Autodesk Inventor part; units mm, degrees
ref_plane "YZ Plane" through (0, 0, 0) normal (1, 0, 0) x (0, 1, 0)
ref_plane "XZ Plane" through (0, 0, 0) normal (0, 1, 0) x (-1, 0, 0)
ref_plane "XY Plane" through (0, 0, 0) normal (0, 0, 1) x (1, 0, 0)
sketch "Drawing" plane through (0, 0, 0) normal (0, 0, 1) x (1, 0, 0)
  line L0 (-58.5227, 93.5052) -> (128.141, 93.5052) construction
  line L1 (128.141, 93.5052) -> (128.141, -71.3811) construction
  line L2 (128.141, -71.3811) -> (-58.5227, -71.3811) construction
  line L3 (-58.5227, -71.3811) -> (-58.5227, 93.5052) construction
  line L4 (-58.5227, 93.5052) -> (-58.5227, 50)
  line L5 (-54.9683, 50) -> (-54.9683, -50)
  line L6 (-58.5227, 50) -> (-54.9683, 50)
  line L7 (0, 0) -> (-54.9683, 0) construction
  line L8 (0, 0) -> (0, 93.5052) construction
  line L9 (0, 93.5052) -> (0, -71.3811)
  line L10 (-58.5227, 0) -> (128.141, 0)
  circle A0 centre (23, 22.25) radius 2.5
  circle A1 centre (23, 22.25) radius 1.5
  circle A2 centre (20, 35) radius 1.75
  dimension "d16" = 164.8863
  dimension "d20" = 3.5544
  dimension "d21" = 100
  dimension "d22" = 43.5052
  dimension "d48" = 5
  dimension "d49" = 1
  dimension "d50" = 3.5
sketch "Sketch2" plane through (0, 0, 0) normal (0, 0, 1) x (1, 0, 0)
  line L0 (28, 50) -> (-28, 50)
  line L1 (-34, 44) -> (-34, -44)
  line L2 (-28, -50) -> (28, -50)
  line L3 (34, -44) -> (34, 44)
  line L4 (34, 50) -> (-34, -50) construction
  line L5 (-34, 50) -> (34, -50) construction
  arc A0 (-28, 50) -> (-34, 44) centre (-28, 44) ccw
  arc A1 (34, 44) -> (28, 50) centre (28, 44) ccw
  arc A2 (-34, -44) -> (-28, -50) centre (-28, -44) ccw
  arc A3 (28, -50) -> (34, -44) centre (28, -44) ccw
  line L6 (28.5085, 38) -> (28.519, 38)
  line L7 (28.0455, -38) -> (28.5, -38)
  line L8 (-58.5227, 0) -> (128.141, 0)
  line L9 (0, 0) -> (0, 93.5052) construction
  line L10 (0, 93.5052) -> (0, -71.3811)
  line L11 (22, 44) -> (22, 44.5)
  line L12 (30.5, 36) -> (30.5, -36)
  line L13 (22.0455, -44) -> (22.0455, -44.5)
  line L14 (-22.0163, -44.039) -> (-22.0163, -44.5)
  line L15 (-30.5, -36.039) -> (-30.5, 36)
  line L16 (-22, 44) -> (-22, 44.5)
  arc A4 (-28, 38) -> (-22, 44) centre (-28, 44) ccw
  arc A5 (22, 44) -> (28, 38) centre (28, 44) ccw
  arc A6 (28.0455, -38) -> (22.0455, -44) centre (28.0455, -44) ccw
  arc A7 (-22.0163, -44.039) -> (-28.0163, -38.039) centre (-28.0163, -44.039) ccw
  arc A8 (-22.0163, -44.5) -> (-20.0163, -46.5) centre (-20.0163, -44.5) ccw
  arc A9 (-30.5, -36.039) -> (-28.5, -38.039) centre (-28.5, -36.039) ccw
  arc A10 (20.0455, -46.5) -> (22.0455, -44.5) centre (20.0455, -44.5) ccw
  arc A11 (28.5, -38) -> (30.5, -36) centre (28.5, -36) ccw
  arc A12 (30.5, 36) -> (28.5, 38) centre (28.5, 36) ccw
  arc A13 (22, 44.5) -> (20, 46.5) centre (20, 44.5) ccw
  arc A14 (-28.5, 38) -> (-30.5, 36) centre (-28.5, 36) ccw
  arc A15 (-20, 46.5) -> (-22, 44.5) centre (-20, 44.5) ccw
  circle A16 centre (23, 22.25) radius 2.5
  circle A17 centre (23, 22.25) radius 1.5
  circle A18 centre (20, 35) radius 1.75
  circle A19 centre (-23, 22.25) radius 2.5
  circle A20 centre (-23, 22.25) radius 1.5
  circle A21 centre (-20, 35) radius 1.75
  circle A22 centre (23, -22.25) radius 2.5
  circle A23 centre (23, -22.25) radius 1.5
  circle A24 centre (20, -35) radius 1.75
  circle A25 centre (-20, -35) radius 1.75
  circle A26 centre (-23, -22.25) radius 2.5
  circle A27 centre (-23, -22.25) radius 1.5
  circle A28 centre (-28, 44) radius 2
  circle A29 centre (28, 44) radius 2
  circle A30 centre (-28, -44) radius 2
  circle A31 centre (28, -44) radius 2
  circle A32 centre (0, 40) radius 2.5
  circle A33 centre (0, 40) radius 1.5
  circle A34 centre (0, -40) radius 2.5
  circle A35 centre (0, -40) radius 1.5
  line L17 (-20.0163, -46.5) -> (20.0455, -46.5)
  line L18 (22, 44.4601) -> (22, 44)
  line L19 (-28, 38) -> (-28.5, 38)
  line L20 (-20, 46.5) -> (20, 46.5)
  line L21 (-28.5, -38.039) -> (-28.5, -38.039)
  line L22 (28.5, 38) -> (28, 38)
  line L23 (-28.493, -38.1054) -> (-28.493, -38.1054)
  line L24 (-28.5, -38.039) -> (-28.0163, -38.039)
  line L25 (23.05, 44) -> (23.05, 44.5)
  arc A36 (23.05, 44.5) -> (20, 47.55) centre (20, 44.5) ccw
  line L26 (20, 47.55) -> (-20, 47.55)
  arc A37 (-20, 47.55) -> (-23.05, 44.5) centre (-20, 44.5) ccw
  line L27 (-23.05, 44.5) -> (-23.05, 44)
  arc A38 (-28, 39.05) -> (-23.05, 44) centre (-28, 44) ccw
  line L28 (-28, 39.05) -> (-28.5, 39.05)
  arc A39 (-28.5, 39.05) -> (-31.55, 36) centre (-28.5, 36) ccw
  line L29 (-31.55, 36) -> (-31.55, -36.039)
  arc A40 (-31.55, -36.039) -> (-28.5, -39.089) centre (-28.5, -36.039) ccw
  line L30 (-28.5, -39.089) -> (-28.0163, -39.089)
  arc A41 (-23.0663, -44.039) -> (-28.0163, -39.089) centre (-28.0163, -44.039) ccw
  line L31 (-23.0663, -44.039) -> (-23.0663, -44.5)
  arc A42 (-23.0663, -44.5) -> (-20.0163, -47.55) centre (-20.0163, -44.5) ccw
  line L32 (-20.0163, -47.55) -> (20.0455, -47.55)
  arc A43 (20.0455, -47.55) -> (23.0955, -44.5) centre (20.0455, -44.5) ccw
  line L33 (23.0955, -44.5) -> (23.0955, -44)
  arc A44 (28.0455, -39.05) -> (23.0955, -44) centre (28.0455, -44) ccw
  line L34 (28.0455, -39.05) -> (28.5, -39.05)
  arc A45 (28.5, -39.05) -> (31.55, -36) centre (28.5, -36) ccw
  line L35 (31.55, -36) -> (31.55, 36)
  arc A46 (31.55, 36) -> (28.5, 39.05) centre (28.5, 36) ccw
  line L36 (28.5, 39.05) -> (28, 39.05)
  arc A47 (23.05, 44) -> (28, 39.05) centre (28, 44) ccw
  line L37 (-33.5, -44) -> (-33.5, 44)
  arc A48 (-28, 49.5) -> (-33.5, 44) centre (-28, 44) ccw
  line L38 (-28, 49.5) -> (28, 49.5)
  arc A49 (33.5, 44) -> (28, 49.5) centre (28, 44) ccw
  line L39 (33.5, 44) -> (33.5, -44)
  arc A50 (28, -49.5) -> (33.5, -44) centre (28, -44) ccw
  line L40 (28, -49.5) -> (-28, -49.5)
  arc A51 (-33.5, -44) -> (-28, -49.5) centre (-28, -44) ccw
  point P0 (-34, 38)
  point P1 (34, 38)
  point P2 (-34, -38)
  point P3 (34, -38)
  point P4 (22, 50)
  point P5 (22, -50)
  point P6 (-34, 46.5)
  point P7 (34, -46.5)
  dimension "OuterWidth" = 68
  dimension "OuterLength" = 100
  dimension "d26" = 6
  dimension "d27" = 6
  dimension "d29" = 6
  dimension "d34" = 6
  dimension "d36" = 2
  dimension "d37" = 6
  dimension "d38" = 6
  dimension "d39" = 6
  dimension "d40" = 6
  dimension "d41" = 11
  dimension "d42" = 27.75
  dimension "d43" = 5
  dimension "d44" = 1
  dimension "d45" = 3.5
  dimension "d46" = 15
  dimension "d47" = 14
  dimension "d52" = 4
  dimension "d53" = 5
  dimension "d54" = 1
  dimension "d55" = 10
  dimension "d56" = 3.5
  dimension "d57" = 3.5
  dimension "d58" = 3.5
  dimension "d59" = 3.5
  dimension "d60" = 6
  dimension "d61" = 6
  dimension "d62" = 6
  dimension "d63" = 6
  dimension "d67" = 1.05
  dimension "d68" = 1.05
  dimension "d86" = 0.5
extrude "SideWalls" add sketch "Sketch2" along normal blind 35 contours A1 L3 L8 L39 A49 L38 L10 L0 | L10 L38 A48 L37 L8 L1 A0 L0 | L38 A49 L39 L8 L35 A46 L36 A47 L25 A36 L26 L10 | L10 L26 A37 L27 A38 L28 A39 L29 L8 L37 A48 L38 | L3 A3 L2 L10 L40 A50 L39 L8 | L26 A36 L25 A47 L36 A46 L35 L8 L12 A12 L6 L22 A5 L11 A13 L20 L10 | L10 L20 A15 L16 A4 L19 A14 L15 L8 L29 A39 L28 A38 L27 A37 L26 | L39 A50 L40 L10 L32 A43 L33 A44 L34 A45 L35 L8 | L8 L37 A51 L40 L10 L2 A2 L1 | L35 A45 L34 A44 L33 A43 L32 L10 L17 A10 L13 A6 L7 A11 L12 L8 | L8 L29 A40 L30 A41 L31 A42 L32 L10 L40 A51 L37 | L8 L15 A9 L24 A7 L14 A8 L17 L10 L32 A42 L31 A41 L30 A40 L29
extrude "GasketRingLower" add sketch "Sketch2" along normal blind 36.85 contours L26 A36 L25 A47 L36 A46 L35 L8 L12 A12 L6 L22 A5 L11 A13 L20 L10 | L10 L20 A15 L16 A4 L19 A14 L15 L8 L29 A39 L28 A38 L27 A37 L26 | L35 A45 L34 A44 L33 A43 L32 L10 L17 A10 L13 A6 L7 A11 L12 L8 | L8 L15 A9 L24 A7 L14 A8 L17 L10 L32 A42 L31 A41 L30 A40 L29
extrude "Bottom" add sketch "Sketch2" along normal blind 2.8 contours A1 L3 L8 L39 A49 L38 L10 L0 | L10 L38 A48 L37 L8 L1 A0 L0 | L38 A49 L39 L8 L35 A46 L36 A47 L25 A36 L26 L10 | L10 L26 A37 L27 A38 L28 A39 L29 L8 L37 A48 L38 | L3 A3 L2 L10 L40 A50 L39 L8 | L26 A36 L25 A47 L36 A46 L35 L8 L12 A12 L6 L22 A5 L11 A13 L20 L10 | L10 L20 A15 L16 A4 L19 A14 L15 L8 L29 A39 L28 A38 L27 A37 L26 | L39 A50 L40 L10 L32 A43 L33 A44 L34 A45 L35 L8 | L8 L37 A51 L40 L10 L2 A2 L1 | L20 A13 L11 A5 L22 A12 L6 L12 L8 L10 A32 | L10 A32 L8 L15 A14 L19 A4 L16 A15 L20 | L35 A45 L34 A44 L33 A43 L32 L10 L17 A10 L13 A6 L7 A11 L12 L8 | L8 L29 A40 L30 A41 L31 A42 L32 L10 L40 A51 L37 | A32 L10 A33 | L10 A33 A32 | L12 A11 L7 A6 L13 A10 L17 L10 A34 L8 | L8 L15 A9 L24 A7 L14 A8 L17 L10 L32 A42 L31 A41 L30 A40 L29 | A33 L10 | L10 A33 | L10 A34 L17 A8 L14 A7 L24 A9 L15 L8 | A34 L10 A35 | L10 A35 A34 | A35 L10 | L10 A35 | A16 | A17 | A18 | A19 | A20 | A21 | A22 | A23 | A24 | A25 | A26 | A27 | A28 | A29 | A30 | A31
extrude "PEMStuds" add sketch "Sketch2" along normal blind 6 contours A32 L10 A33 | L10 A33 A32 | A33 L10 | L10 A33 | A34 L10 A35 | L10 A35 A34 | A35 L10 | L10 A35 | A16 | A17 | A19 | A20 | A22 | A23 | A26 | A27
extrude "SmallerSupports" add sketch "Sketch2" along normal blind 4 contours A18 | A21 | A24 | A25
sketch "Sketch4" plane through (-23, -22.25, 6) normal (0, 0, 1) x (1, 0, 0)
  circle A0 centre (23, -17.75) radius 2.5
  circle A1 centre (46, 0) radius 2.5
  circle A2 centre (23, 62.25) radius 2.5
  circle A3 centre (0, 0) radius 2.5
  circle A4 centre (46, 44.5) radius 2.5
  circle A5 centre (-5, -21.75) radius 2
  circle A6 centre (51, -21.75) radius 2
  circle A7 centre (-5, 66.25) radius 2
  circle A8 centre (51, 66.25) radius 2
  circle A9 centre (0, 44.5) radius 2.5
  point P0 (23, 22.25)
  dimension "d101" = 17.75
  dimension "d102" = 23
hole "PEMStudHoles" at (0, -40, 6) at (23, -22.25, 6) at (0, 40, 6) at (-23, -22.25, 6) at (23, 22.25, 6) at (-23, 22.25, 6) direction (0, 0, -1) diameter 3 depth 4
hole "Hole2" at (28, 44, 6) at (-28, 44, 6) at (-28, -44, 6) at (28, -44, 6) direction (0, 0, -1) diameter 6 end through all both
ref_plane "Work Plane2" through (-32.2426, 48.2426, 35) normal (0, 0, 1) x (1, 0, 0)
sketch "Sketch6" plane through (-32.2426, 48.2426, 35) normal (0, 0, 1) x (1, 0, 0)
  line L0 (-1.2574, -92.2426) -> (-1.2574, -4.2426)
  arc A0 (4.2426, 1.2574) -> (-1.2574, -4.2426) centre (4.2426, -4.2426) ccw
  line L1 (4.2426, 1.2574) -> (60.2426, 1.2574)
  arc A1 (65.7426, -4.2426) -> (60.2426, 1.2574) centre (60.2426, -4.2426) ccw
  line L2 (65.7426, -4.2426) -> (65.7426, -92.2426)
  arc A2 (60.2426, -97.7426) -> (65.7426, -92.2426) centre (60.2426, -92.2426) ccw
  line L3 (60.2426, -97.7426) -> (4.2426, -97.7426)
  arc A3 (-1.2574, -92.2426) -> (4.2426, -97.7426) centre (4.2426, -92.2426) ccw
  line L4 (-1.7574, -4.2426) -> (-1.7574, -92.2426)
  arc A4 (-1.7574, -92.2426) -> (4.2426, -98.2426) centre (4.2426, -92.2426) ccw
  line L5 (4.2426, -98.2426) -> (60.2426, -98.2426)
  arc A5 (60.2426, -98.2426) -> (66.2426, -92.2426) centre (60.2426, -92.2426) ccw
  line L6 (66.2426, -92.2426) -> (66.2426, -4.2426)
  arc A6 (66.2426, -4.2426) -> (60.2426, 1.7574) centre (60.2426, -4.2426) ccw
  line L7 (60.2426, 1.7574) -> (4.2426, 1.7574)
  arc A7 (4.2426, 1.7574) -> (-1.7574, -4.2426) centre (4.2426, -4.2426) ccw
  line L8 (4.2426, 1.2574) -> (60.2426, 1.2574)
  arc A8 (65.7426, -4.2426) -> (60.2426, 1.2574) centre (60.2426, -4.2426) ccw
  line L9 (65.7426, -4.2426) -> (65.7426, -92.2426)
  arc A9 (60.2426, -97.7426) -> (65.7426, -92.2426) centre (60.2426, -92.2426) ccw
  line L10 (60.2426, -97.7426) -> (4.2426, -97.7426)
  arc A10 (-1.2574, -92.2426) -> (4.2426, -97.7426) centre (4.2426, -92.2426) ccw
  line L11 (-1.2574, -92.2426) -> (-1.2574, -4.2426)
  arc A11 (4.2426, 1.2574) -> (-1.2574, -4.2426) centre (4.2426, -4.2426) ccw
  point P0 (32.2426, -48.2426)
  dimension "d97" = 0.5
  dimension "d98" = 0.5
extrude "Extrusion8" cut sketch "Sketch6" against normal blind 0.5
equation "\"d16\" = 28.0458 * ImageScale"
equation "\"d20\" = 0.604577 * ImageScale"
equation "\"d21\" = 17.0092 * ImageScale"
equation "\"d22\" = 7.39989 * ImageScale"
equation "\"d29\" = OuterFillet"
equation "\"d37\" = OuterFillet"
equation "\"d38\" = OuterFillet"
equation "\"d39\" = OuterFillet"
equation "\"d40\" = OuterFillet"
equation "\"ImageScale\" = 0.587917"
equation "\"WallThickness\" = 3.5"
equation "\"OuterFillet\" = 6"
properties part number "PinfoxBox" material "Polypropylene"
Design review of the part built by this model. Coordinates are the model's own, in mm. A direction names the side the tool comes from. Coordinates: 2 decimals unless noted, no trailing zeros. Loops run counter-clockwise (first coordinate to the right, second up) from the corner with the lowest first, then second, coordinate; pieces in that order, holes last. Notation, with made-up numbers: (11, 6) - (19, 6) arc R10 cw to (19, 11) - close; hole circle Ø9 at (59.25, 9). An arc over 180 degrees is marked (long way). Use CSV: the item, a comma, the result in double quotes. Start each with the question number.
1) Tool access review of faces 4 (the cylindrical face through (28, 47, 17)), 5 (the cylindrical face through (-24.84, -23.94, 4.38)), 6 (the cylindrical face through (-31.93, -47.85, 34.75)): name each direction out of +Z, -Z, +X, -X, +Y, -Y from which nothing blocks a thin tool from reaching the whole face with its end or side.
2) For pin 1 Ø2 at (x, y) = (-8, -33) entering from +Z; pin 2 Ø6 at (x, y) = (9, 16.5) entering from -Z; pin 3 Ø0.9 at (x, y) = (23.5, -21.5) entering from +Z; pin 4 Ø0.5 at (x, z) = (-28.5, 36) entering from -Y, all flat-tipped, find the tip position at first contact; note any pin that passes through.
3) Consider section B-B on x = 5.5. Write out the cut boundary in (y, z).
4) Wall thickness on L1, parallel to Y at x = 28, z = 16.5; L2, parallel to X at y = 44, z = 22.5; L3, parallel to Y at x = -12, z = 5: over which ranges is each line inside the solid? List them lowest first. Write a range as from..to.
5) Consider section D-D on y = 7.5. Write out the cut boundary in (x, z), then the cut area to 3 significant figures.
6) Consider section C-C on z = 13. Give the number of separate pieces and of enclosed holes in the cut face, then the cut area to 3 significant figures.
7) The part is to be moulded in two halves that separate along Y. For faces 1 (the cylindrical face through (-21.39, -33.94, 3.39)), 2 (the cylindrical face through (-31.85, 47.93, 34.75)), 3 (the flat face through (0, -50, 17)), say which applies: +Y half, -Y half, draft (parallel to the pull), parting line (faces both ways), or undercut.
Geometry says:
1,face 4,"+Z, -Z"
1,face 5,"+Z"
1,face 6,"+Z, -X, -Y"
2,pin 1,"z = 2.8"
2,pin 2,"z = 0"
2,pin 3,"z = 2"
2,pin 4,"y = -39.09"
3,outline,"(-50, 0) - (50, 0) - (50, 34.5) - (49.5, 34.5) - (49.5, 35) - (47.55, 35) - (47.55, 36.85) - (46.5, 36.85) - (46.5, 2.8) - (-46.5, 2.8) - (-46.5, 36.85) - (-47.55, 36.85) - (-47.55, 35) - (-49.5, 35) - (-49.5, 34.5) - (-50, 34.5) - close"
4,L1,"-50..-47, -41..-38, 38..41, 47..50"
4,L2,"-34..-31, -25..-22, 22..25, 31..34"
4,L3,"-50..-46.5, 46.5..50"
5,outline,"(-34, 0) - (34, 0) - (34, 34.5) - (33.5, 34.5) - (33.5, 35) - (31.55, 35) - (31.55, 36.85) - (30.5, 36.85) - (30.5, 2.8) - (-30.5, 2.8) - (-30.5, 36.85) - (-31.55, 36.85) - (-31.55, 35) - (-33.5, 35) - (-33.5, 34.5) - (-34, 34.5) - close"
5,area,"419 mm^2"
6,separate pieces,"1"
6,enclosed holes,"5"
6,area,"1,250 mm^2"
7,face 1,"undercut"
7,face 2,"+Y half"
7,face 3,"-Y half"
